Drawing for the job (mm, zero at the part's lowest x, y, z). A direction names the side the tool comes from. Coordinates: 2 decimals unless noted, no trailing zeros. Write each loop counter-clockwise with the first axis right and the second up, starting at its lowest first coordinate (ties: lowest second). Pieces come first, ordered by that corner, then holes. Notation, with made-up numbers: M 62,24.5 L 92,24.5 A14 cw 92,43.5 Z; hole C 56,-33.5 d9. An arc over 180 degrees is marked long. Put each result on its own line as item: value. Start each with the question number.
Q1. Cut at B-B (x = 16). Write the cut outline in (y, z), then the cut area to 3 significant figures.
Q2. Which spindle directions (+Z, -Z, +X, -X, +Y, -Y) get a long thin tool onto all of the face, cutting with end or side? Do the marked faces 1, 2 and 3. Say none if no direction does.
Q3. Drill centre lines: line 1 along Z through (x, y) = (20, 22); line 2 along Y through (x, z) = (3.5, 3.5); line 3 along Y through (x, z) = (25, 22.5). Where is each one in solid material? Low to high.
Q4. Drop flat-ended pins along their axis: pin 1 (1.5 mm diameter, centred on x = 16, y = 5.5, fed in from +Z); pin 2 (9 mm diameter, centred on x = 8, z = 5, fed in from -Y); pin 3 (6 mm diameter, centred on x = 17, z = 24.5, fed in from -Y). Give the stop position or say it passes through.
Q5. Cut at A-A (y = 35.5). Write the cut outline in (x, z), then the cut area to 3 significant figures.
Q6. Cut at D-D (z = 14.75). Write the cut outline in (x, y).
Q7. Cut at C-C (z = 10). Write the cut outline in (x, y).
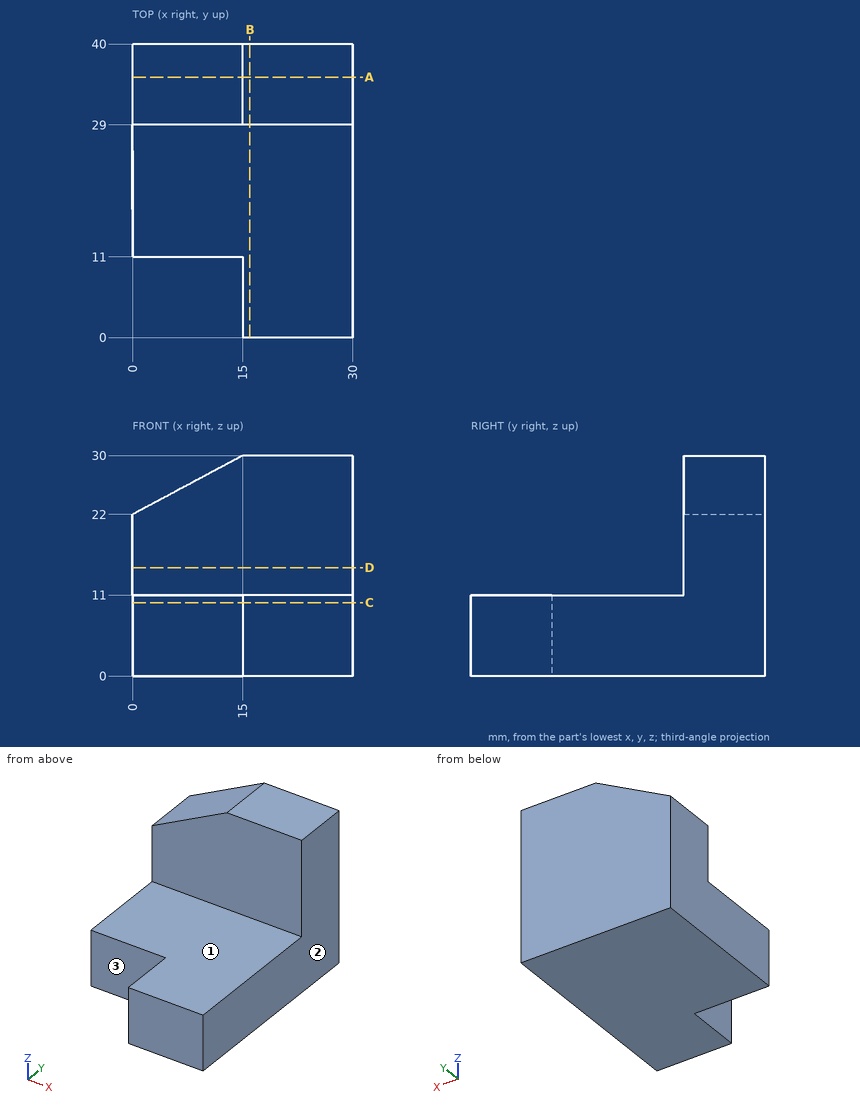
Computed values:
1. outline: M 0,0 L 40,0 L 40,30 L 29,30 L 29,11 L 0,11 Z
1. area: 649 mm2
2. face 1: +Z, +X, -X, -Y
2. face 2: +Z, -Z, +X, +Y, -Y
2. face 3: +Z, -Z, -X, -Y
3. line 1: 0 to 11
3. line 2: 11 to 40
3. line 3: 29 to 40
4. pin 1: z = 11
4. pin 2: y = 11
4. pin 3: y = 29
5. outline: M 0,0 L 30,0 L 30,30 L 15,30 L 0,22 Z
5. area: 840 mm2
6. outline: M 0,29 L 30,29 L 30,40 L 0,40 Z
7. outline: M 0,11 L 15,11 L 15,0 L 30,0 L 30,40 L 0,40 Z
